```python
from build123d import *

# Parameters (mm, degrees)
SKETCH1_R           = 17.5
SKETCH1_R_2         = 1.5
BOSS_EXTRUDE1_DEPTH = 5
SKETCH3_R           = 1.5
BOSS_EXTRUDE2_DEPTH = 5
SKETCH4_W           = 35
SKETCH4_H           = 54
BOSS_EXTRUDE3_DEPTH = 5
FILLET1_R           = 10
SKETCH6_W           = 35
SKETCH6_H           = 12
BOSS_EXTRUDE4_DEPTH = 120
CUT_EXTRUDE1_REACH  = 35
SKETCH7_R           = 1.3
SKETCH7_W           = 21
SKETCH7_H           = 41
CUT_EXTRUDE2_DEPTH  = 12
LPATTERN1_COUNT     = 3
LPATTERN1_PITCH     = 16
FILLET2_R           = 10
FILLET3_R           = 2
SKETCH11_R          = 0.7
SKETCH11_R_2        = 1.5
CUT_EXTRUDE3_DEPTH  = 55
SKETCH12_R          = 2.5
CUT_EXTRUDE4_DEPTH  = 2
SKETCH13_R          = 2.5
CUT_EXTRUDE5_DEPTH  = 2


with BuildPart() as part:
    # Sketch1 → Boss-Extrude1 (new body)
    with BuildSketch(Plane(origin=(0, 0, 0), x_dir=(1, 0, 0), z_dir=(0, 1, 0))):
        Circle(SKETCH1_R)
        Circle(SKETCH1_R_2, mode=Mode.SUBTRACT)
        with BuildLine():
            Line((-17.5, 20), (-17.5, 0))
            ThreePointArc((-17.5, 0), (0, 17.5), (17.5, 0))
            Line((17.5, 0), (17.5, 20))
            Line((17.5, 20), (-17.5, 20))
        make_face()
    extrude(amount=BOSS_EXTRUDE1_DEPTH)



with BuildPart() as body_2:
    # Sketch3 → Boss-Extrude2 (new body)
    with BuildSketch(Plane(origin=(0, -49, 0), x_dir=(1, 0, 0), z_dir=(0, 1, 0))):
        with BuildLine():
            Line((17.5, 0), (17.5, 20))
            Line((17.5, 20), (-17.5, 20))
            Line((-17.5, 20), (-17.5, 0))
            ThreePointArc((-17.5, 0), (0, -17.5), (17.5, 0))
        make_face()
        Circle(SKETCH3_R, mode=Mode.SUBTRACT)
    extrude(amount=BOSS_EXTRUDE2_DEPTH)


with BuildPart() as part_1:
    add(part.part)

    add(body_2.part)  # Boss-Extrude3 merges body 2
    # Sketch4 → Boss-Extrude3 (add)
    with BuildSketch(Plane(origin=(0, 0, -20), x_dir=(-1, 0, 0), z_dir=(0, 0, -1))):
        with Locations((0, -22)):
            Rectangle(SKETCH4_W, SKETCH4_H)
    extrude(amount=BOSS_EXTRUDE3_DEPTH)

    # Fillet1
    fillet1_edges = [part_1.edges().sort_by_distance(p)[0] for p in [
        (0, -49, -25),
        (0, 5, -25),
        (0, -44, -20),
        (0, 0, -20),
    ]]
    fillet(fillet1_edges, radius=FILLET1_R)

    # Sketch6 → Boss-Extrude4 (add)
    with BuildSketch(Plane(origin=(0, 0, -25), x_dir=(-1, 0, 0), z_dir=(0, 0, -1))):
        with Locations((0, -22)):
            Rectangle(SKETCH6_W, SKETCH6_H)
    extrude(amount=BOSS_EXTRUDE4_DEPTH)

    # Sketch7 → Cut-Extrude1 (cut, up to next)
    with BuildSketch(Plane(origin=(0, -16, 0), x_dir=(1, 0, 0), z_dir=(0, 1, 0)), mode=Mode.PRIVATE) as cut_extrude1_sk1:
        with Locations((-5, 140.5)):
            Circle(SKETCH7_R)
    cut_extrude1_tool1 = extrude(cut_extrude1_sk1.sketch, amount=-CUT_EXTRUDE1_REACH, mode=Mode.PRIVATE) & part_1.part
    add(cut_extrude1_tool1.solids().sort_by_distance((-5, -16, -140.5))[0], mode=Mode.SUBTRACT)
    # Sketch7 → Cut-Extrude1 (cut, up to next)
    with BuildSketch(Plane(origin=(0, -16, 0), x_dir=(1, 0, 0), z_dir=(0, 1, 0)), mode=Mode.PRIVATE) as cut_extrude1_sk2:
        with Locations((5, 140.5)):
            Circle(SKETCH7_R)
    cut_extrude1_tool2 = extrude(cut_extrude1_sk2.sketch, amount=-CUT_EXTRUDE1_REACH, mode=Mode.PRIVATE) & part_1.part
    add(cut_extrude1_tool2.solids().sort_by_distance((5, -16, -140.5))[0], mode=Mode.SUBTRACT)
    # Sketch7 → Cut-Extrude1 (cut, up to next)
    with BuildSketch(Plane(origin=(0, -16, 0), x_dir=(1, 0, 0), z_dir=(0, 1, 0)), mode=Mode.PRIVATE) as cut_extrude1_sk3:
        with Locations((5, 92.5)):
            Circle(SKETCH7_R)
    cut_extrude1_tool3 = extrude(cut_extrude1_sk3.sketch, amount=-CUT_EXTRUDE1_REACH, mode=Mode.PRIVATE) & part_1.part
    add(cut_extrude1_tool3.solids().sort_by_distance((5, -16, -92.5))[0], mode=Mode.SUBTRACT)
    # Sketch7 → Cut-Extrude1 (cut, up to next)
    with BuildSketch(Plane(origin=(0, -16, 0), x_dir=(1, 0, 0), z_dir=(0, 1, 0)), mode=Mode.PRIVATE) as cut_extrude1_sk4:
        with Locations((-5, 92.5)):
            Circle(SKETCH7_R)
    cut_extrude1_tool4 = extrude(cut_extrude1_sk4.sketch, amount=-CUT_EXTRUDE1_REACH, mode=Mode.PRIVATE) & part_1.part
    add(cut_extrude1_tool4.solids().sort_by_distance((-5, -16, -92.5))[0], mode=Mode.SUBTRACT)
    # Sketch7 → Cut-Extrude1 (cut, up to next)
    with BuildSketch(Plane(origin=(0, -16, 0), x_dir=(1, 0, 0), z_dir=(0, 1, 0)), mode=Mode.PRIVATE) as cut_extrude1_sk5:
        with Locations((0, 116.5)):
            Rectangle(SKETCH7_W, SKETCH7_H)
    cut_extrude1_tool5 = extrude(cut_extrude1_sk5.sketch, amount=-CUT_EXTRUDE1_REACH, mode=Mode.PRIVATE) & part_1.part
    add(cut_extrude1_tool5.solids().sort_by_distance((0, -16, -116.5))[0], mode=Mode.SUBTRACT)

    # Sketch8 → Cut-Extrude2 (cut)
    with BuildSketch(Plane(origin=(0, -16, 0), x_dir=(1, 0, 0), z_dir=(0, 1, 0))):
        Polygon((10.5, 84), (-10.5, 84), (-10.5, 74.207539179), align=None)
        Polygon((10.5, 71.207539179), (10.5, 81), (-10.5, 71.207539179), align=None)
    cut_extrude2 = extrude(amount=-CUT_EXTRUDE2_DEPTH, mode=Mode.SUBTRACT)

    # LPattern1: Cut-Extrude2 ×3
    with Locations(*[(0, 0, i * LPATTERN1_PITCH) for i in range(1, LPATTERN1_COUNT)]):
        add(cut_extrude2, mode=Mode.SUBTRACT)

    # Fillet2
    fillet2_edges = [part_1.edges().sort_by_distance(p)[0] for p in [
        (0, -28, -25),
        (0, -16, -25),
    ]]
    fillet(fillet2_edges, radius=FILLET2_R)

    # Fillet3
    fillet3_edges = [part_1.edges().sort_by_distance(p)[0] for p in [
        (17.5, -22, -145),
        (0, -28, -145),
        (-17.5, -22, -145),
        (0, -16, -145),
    ]]
    fillet(fillet3_edges, radius=FILLET3_R)

    # Sketch11 → Cut-Extrude3 (cut, through all)
    with BuildSketch(Plane(origin=(0, 5, 0), x_dir=(1, 0, 0), z_dir=(0, 1, 0))):
        with Locations((0, 7.2)):
            Circle(SKETCH11_R)
        Circle(SKETCH11_R_2)
        with Locations((0, -7.2)):
            Circle(SKETCH11_R)
    extrude(amount=-CUT_EXTRUDE3_DEPTH, mode=Mode.SUBTRACT)

    # Sketch12 → Cut-Extrude4 (cut)
    with BuildSketch(Plane.XZ):
        Circle(SKETCH12_R)
    extrude(amount=-CUT_EXTRUDE4_DEPTH, mode=Mode.SUBTRACT)

    # Sketch13 → Cut-Extrude5 (cut)
    with BuildSketch(Plane(origin=(0, -44, 0), x_dir=(1, 0, 0), z_dir=(0, 1, 0))):
        Circle(SKETCH13_R)
    extrude(amount=-CUT_EXTRUDE5_DEPTH, mode=Mode.SUBTRACT)


solid = part_1.part
```
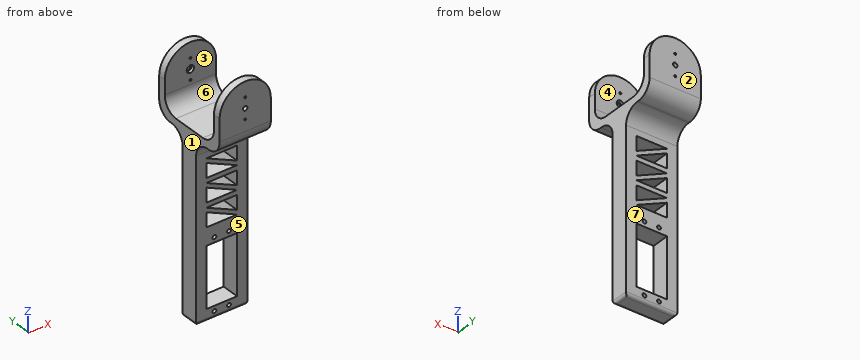
Read the model definition and answer for the solid it produces. Units are mm, in the model's axes. Face numbers are marked on the shaded views. A direction names the side the tool comes from. Round coordinates to 2 decimals unless told otherwise and drop trailing zeros. Write each loop counter-clockwise with the first axis right and the second up, starting at its lowest first coordinate (ties: lowest second). Pieces come first, ordered by that corner, then holes. Notation, with made-up numbers: (64, 88.25) - (71, 88.25) arc R23 cw to (71, 100.25) - close; hole circle Ø5 at (86, 37). An arc over 180 degrees is marked (long way). One line per item, written item: value.
Q1. Find section A-A (y = -20.5). Count the separate pieces of the cut face and the enclosed holes in it, and give its area (3 significant figures).
The answers:
separate pieces: 1
enclosed holes: 11
area: 2,870 mm2
Q2. Find section B-B (x = 12.5). Determine the outline of the cut face in (y, z), and give its area (3 significant figures).
The answers:
outline: (-49, -15) arc R10 ccw to (-39, -25) - (-38, -25) arc R10 cw to (-28, -35) - (-28, -143) arc R2 ccw to (-26, -145) - (-18, -145) arc R2 ccw to (-16, -143) - (-16, -35) arc R10 cw to (-6, -25) - (-5, -25) arc R10 ccw to (5, -15) - (5, 12.25) - (0, 12.25) - (0, -10) arc R10 cw to (-10, -20) - (-34, -20) arc R10 cw to (-44, -10) - (-44, 12.25) - (-49, 12.25) - close
area: 2,070 mm2
Q3. Find section C-C (z = -32.5). Determine the outline of the cut face in (x, y).
The answers:
outline: (-17.5, -28.32) - (17.5, -28.32) - (17.5, -15.68) - (-17.5, -15.68) - close
Q4. Find section D-D (y = -1.5). Determine the outline of the cut face in (x, z), and give its area (3 significant figures).
The answers:
outline: (-17.5, -24.37) - (17.5, -24.37) - (17.5, -15.27) - (-17.5, -15.27) - close
area: 318 mm2
Q5. Each of these flat-tipped pins is pushed along its axis until it touches: P1, Ø6, axis at x = 4.5, y = -23, coming from the +Z side; P2, Ø1.1, axis at x = 7.5, y = -5.5, coming from the -Z side; P3, Ø2.5, axis at x = -0.5, z = 1, coming from the +Y side; P4, Ø3, axis at x = 5, z = -92.5, coming from the +Y side. Where does it stop, or does it pass through?
The answers:
P1: stops at z = -20
P2: stops at z = -25
P3: stops at y = 5
P4: stops at y = -16
Q6. Straight lines are drawn through the part: line 1 (Y direction, x = 16, z = -5); line 2 (Z direction, x = 0, y = -45.3); line 3 (Z direction, x = 0, y = 1). For each, find the intervals that lie inside material, in ascending order. Write a range as from..to.
The answers:
line 1: y = -49..-44, 0..5
line 2: z = -22.77..-7.9, -6.5..-2.5, 2.5..6.5, 7.9..17.5
line 3: z = -23..-7.9, -6.5..-2.5, 2.5..6.5, 7.9..17.5
Q7. Which of the six approach directions +Z, -Z, +X, -X, +Y, -Y give full straight-line access (tool end or side, diameter ignored) to the marked faces 5, 6 and 7?
The answers:
face 5: -Z, +X, -X, -Y
face 6: +Z, +X, -X
face 7: -Z, +X, -X, +Y
Q8. For a pull along Y with two mould halves and no side action, classify the marked faces 1, 2, 3 and 4 as pulls with the +Y half, pulls with the -Y half, needs draft (parallel to the pull), parting line crosses it, or undercut.
The answers:
face 1: needs draft
face 2: pulls with the +Y half
face 3: undercut
face 4: undercut
